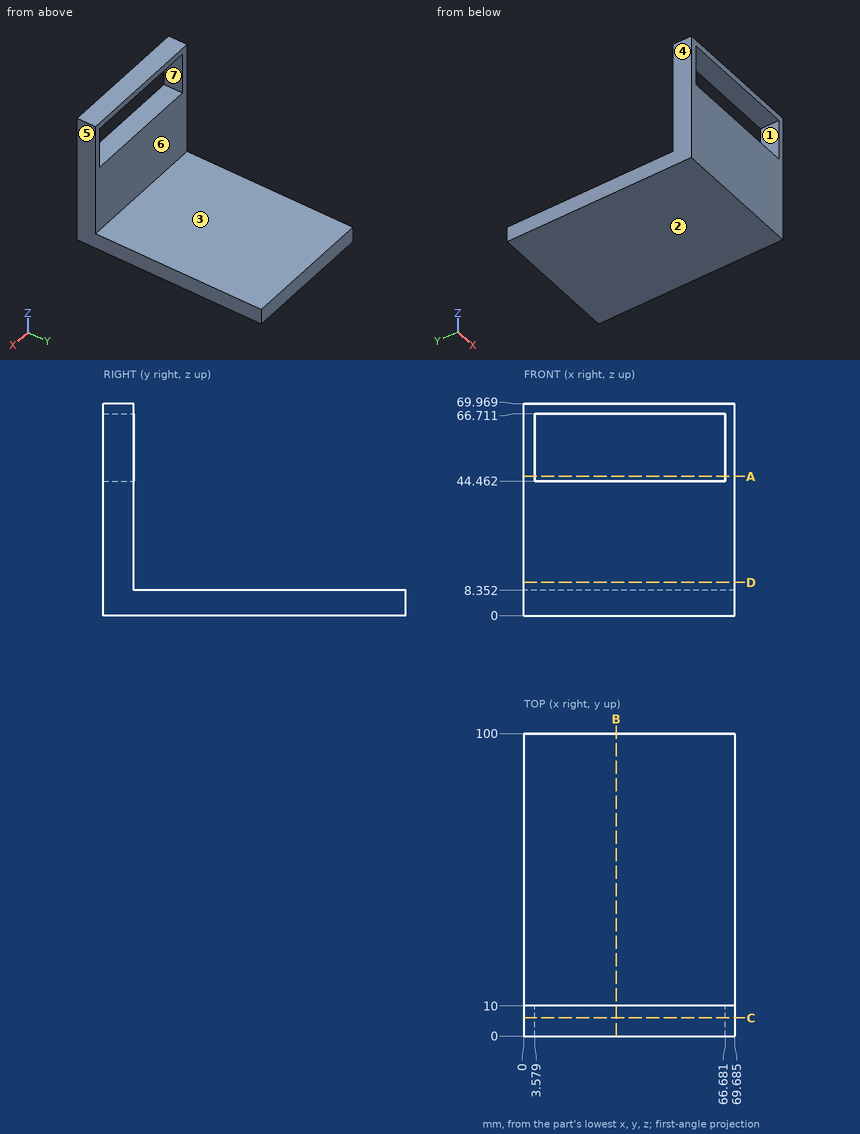
Job drawing, mm, ordinate dimensions from the low corner. One solid piece. A direction names the side the tool comes from. Coordinates: 2 decimals unless noted, no trailing zeros. Order: outer loops, then holes, each group sorted by start corner. A loop starts at its lowest first (then second) coordinate and runs counter-clockwise, first axis right, second up. Notation, with made-up numbers: (41, 1.25) - (96, 1.25) arc R15 cw to (96, 19.25) - close; hole circle Ø5 at (-31, -32.5). An arc over 180 degrees is marked (long way). Write each question's results on one line, items separated by ' | '. Start each with the question number.
Item 1: Flat gauge pins, fed straight in: pin 1 (10 mm diameter, centred on x = 42.5, y = 26, fed in from +Z); pin 2 (8 mm diameter, centred on y = 4, z = 50, fed in from -X); pin 3 (10 mm diameter, centred on x = 47.5, z = 46.5, fed in from +Y). Where does each tip first touch, or does it go through?
Item 2: Mould opens along Z. For the marked faces 1, 2, 3 and 4 say: released by +Z, released by -Z, zero draft, split by the parting line, or undercut.
Item 3: Band-saw the part on B-B on x = 30.5. Write the cut outline in (y, z), and give its area (3 significant figures).
Item 4: Band-saw the part on A-A on z = 46. Write the cut outline in (x, y) (1 decimal).
Item 5: Band-saw the part on C-C on y = 6. Write the cut outline in (x, z) (1 decimal), and give its area (3 significant figures).
Item 6: Band-saw the part on D-D on z = 11. Write the cut outline in (x, y) (1 decimal), and give its area (3 significant figures).
Item 7: Tool access for the marked faces 5, 6 and 7: list every direction of +Z, -Z, +X, -X, +Y, -Y with a clear straight run to the whole face (end or side of a thin tool).
Item 8: Wall check: probe 1 along Y at (x, z) = (10, 20); probe 2 along Z at (x, y) = (8, 19.5). Give the ranges that are in metal, low to high. Write a range as [from, to].
Numbers:
1) pin 1: z = 8.35 | pin 2: x = 0 | pin 3: y = 10
2) face 1: undercut | face 2: released by -Z | face 3: released by +Z | face 4: zero draft
3) outline: (0, 0) - (100, 0) - (100, 8.35) - (10, 8.35) - (10, 44.46) - (0, 44.46) - close; (0, 66.71) - (10, 66.71) - (10, 69.97) - (0, 69.97) - close | area: 1,230 mm^2
4) outline: (0, 0) - (3.6, 0) - (3.6, 10) - (0, 10) - close; (66.7, 0) - (69.7, 0) - (69.7, 10) - (66.7, 10) - close
5) outline: (0, 0) - (69.7, 0) - (69.7, 70) - (0, 70) - close; hole (3.6, 44.5) - (66.7, 44.5) - (66.7, 66.7) - (3.6, 66.7) - close | area: 3,470 mm^2
6) outline: (0, 0) - (69.7, 0) - (69.7, 10) - (0, 10) - close | area: 697 mm^2
7) face 5: +Z, -Z, +X, +Y, -Y | face 6: +Z, +X, -X, +Y | face 7: +Y, -Y
8) probe 1: [0, 10] | probe 2: [0, 8.35]
